```python
from build123d import *

# Parameters (mm, degrees)
SKETCH1_W           = 160
SKETCH1_H           = 65
BOSS_EXTRUDE1_DEPTH = 36
SKETCH2_R           = 3.175
BOSS_EXTRUDE3_DEPTH = 12.7
FILLET1_R           = 7.62


with BuildPart() as part:
    # Sketch1 → Boss-Extrude1 (new body)
    with BuildSketch(Plane(origin=(0, 0, 0), x_dir=(1, 0, 0), z_dir=(0, 1, 0))):
        with Locations((38.916030534, -15.255725191)):
            Rectangle(SKETCH1_W, SKETCH1_H)
    extrude(amount=BOSS_EXTRUDE1_DEPTH)

    # Sketch2 → Boss-Extrude3 (add)
    with BuildSketch(Plane(origin=(118.916030534, 0, 0), x_dir=(0, 0, -1), z_dir=(1, 0, 0))):
        with Locations(Location((-44.580725191, 21.4925, 0), (0, 0, 180))):
            Circle(SKETCH2_R)
        with Locations(Location((-44.580725191, 14.5075, 0), (0, 0, 180))):
            Circle(SKETCH2_R)
    extrude(amount=BOSS_EXTRUDE3_DEPTH)

    # Fillet1
    fillet1_edges = [part.edges().sort_by_distance(p)[0] for p in [
        (118.916030534, 36, 15.255725191),
        (38.916030534, 36, -17.244274809),
        (-41.083969466, 36, 15.255725191),
        (38.916030534, 0, -17.244274809),
        (118.916030534, 0, 15.255725191),
        (38.916030534, 0, 47.755725191),
        (-41.083969466, 0, 15.255725191),
        (38.916030534, 36, 47.755725191),
    ]]
    fillet(fillet1_edges, radius=FILLET1_R)


solid = part.part
```
Input: part model. Units: mm. Frame: model coordinates. Round coordinates to 2 decimals unless told otherwise and drop trailing zeros. Order: outer loops, then holes, each group sorted by start corner. A loop starts at its lowest first (then second) coordinate and runs counter-clockwise, first axis right, second up. Notation, with made-up numbers: (-14.5, 84.25) - (-0.5, 84.25) arc R3 ccw to (-0.5, 89.25) - close; hole circle Ø8 at (28.25, 23). An arc over 180 degrees is marked (long way). One line per question, with ' | ' between items. Start each with the question number.
1) Ray query, probe 1 along X at (y, z) = (7, -4); probe 2 along Z at (x, y) = (-4, 28.5); probe 3 along Z at (x, y) = (109, 30.5). Return the intervals inside material, ascending.
2) Pull-direction query (Y, two-part tool) for faces 1 (the cylindrical face through (116.62, 33.83, 14.8)), 2 (the cylindrical face through (116.62, 2.17, 14.8)), 3 (the cylindrical face through (125.18, 13.55, 47.61)), 4 (the cylindrical face through (125.177, 22.709, 47.514)); classes: +Y half, -Y half, draft (parallel to the pull), parting line (faces both ways), or undercut.
3) Cut plane A-A, the plane z = 27.5. Return the cut outline in (x, y), then the cut area to 3 significant figures.
4) Contact query for a flat-ended pin moving along its axis: P1, Ø10.5, axis at y = 19, z = 26.5, coming from the +X side. Output: stop coordinate, or through.
5) Cut plane C-C, the plane y = 30. Return the cut outline in (x, z).
6) Cut plane B-B, the plane x = 81. Return the cut outline in (y, z).
Worked out:
1) probe 1: x = -41.06 to 118.89 | probe 2: z = -17.24 to 47.75 | probe 3: z = -16.94 to 47.45
2) face 1: +Y half | face 2: -Y half | face 3: undercut | face 4: undercut
3) outline: (-41.08, 7.62) arc R7.62 ccw to (-33.46, 0) - (111.3, 0) arc R7.62 ccw to (118.92, 7.62) - (118.92, 28.38) arc R7.62 ccw to (111.3, 36) - (-33.46, 36) arc R7.62 ccw to (-41.08, 28.38) - close | area: 5,710 mm^2
4) P1: stops at x = 118.92
5) outline: (-40.91, -17.07) - (118.74, -17.07) - (118.74, 47.58) - (-40.91, 47.58) - close
6) outline: (0, -9.62) arc R7.62 ccw to (7.62, -17.24) - (28.38, -17.24) arc R7.62 ccw to (36, -9.62) - (36, 40.14) arc R7.62 ccw to (28.38, 47.76) - (7.62, 47.76) arc R7.62 ccw to (0, 40.14) - close
